```python
from build123d import *

# Parameters (mm, degrees)
F0_W      = 42
F0_H      = 63
F0_R      = 1.75
F0_R_2    = 11.5
F1_DEPTH  = 4
F2_W      = 42
F2_H      = 3
F3_DEPTH  = 30
F4_R      = 2.876713
F4_R_2    = 4.342344
F4_R_3    = 6.646556
F5_DEPTH  = 4
F6_W      = 3
F6_H      = 10
F7_DEPTH  = 10
F8_R      = 2
F9_DEPTH  = 25
F10_W     = 3
F10_H     = 34
F11_DEPTH = 10
F12_R     = 2
F13_DEPTH = 25


with BuildPart() as f1:
    # F0 (on Top) → F1 (new body)
    with BuildSketch(Plane.XY):
        Rectangle(F0_W, F0_H)
        with Locations((-15.5, -5)):
            Circle(F0_R, mode=Mode.SUBTRACT)
        with Locations((15.5, -5)):
            Circle(F0_R, mode=Mode.SUBTRACT)
        with Locations((-15.5, 26)):
            Circle(F0_R, mode=Mode.SUBTRACT)
        with Locations((0, 10.5)):
            Circle(F0_R_2, mode=Mode.SUBTRACT)
        with Locations((15.5, 26)):
            Circle(F0_R, mode=Mode.SUBTRACT)
    extrude(amount=F1_DEPTH)

    # F2 (on face) → F3 (join)
    with BuildSketch(Plane.XY.offset(4)):
        with Locations((0, -30)):
            Rectangle(F2_W, F2_H)
    extrude(amount=F3_DEPTH)

    # F4 (on face) → F5 (join)
    with BuildSketch(Plane(origin=(-21, 0, 0), x_dir=(0, -1, 0), z_dir=(-1, 0, 0))):
        Polygon((28.5, 34), (-31.5, 4), (28.5, 4), align=None)
        with Locations((-5.90477, 9.762893)):
            Circle(F4_R, mode=Mode.SUBTRACT)
        with Locations((4.623126, 12.472619)):
            Circle(F4_R_2, mode=Mode.SUBTRACT)
        with Locations((19.102728, 16.427787)):
            Circle(F4_R_3, mode=Mode.SUBTRACT)
        Polygon((28.5, 4), (-31.5, 4), (-31.5, 0), (31.5, 0), (31.5, 34), (28.5, 34), align=None)
    extrude(amount=F5_DEPTH)

    # F6 (on face) → F7 (join)
    with BuildSketch(Plane.YZ.offset(21)):
        with Locations((-30, 29)):
            Rectangle(F6_W, F6_H)
    extrude(amount=F7_DEPTH)

    # F8 (on face) → F9 (cut)
    with BuildSketch(Plane(origin=(0, -28.5, 0), x_dir=(-1, 0, 0), z_dir=(0, 1, 0))):
        with Locations((-26.502214, 29.595299)):
            Circle(F8_R)
    extrude(amount=-F9_DEPTH, mode=Mode.SUBTRACT)

    # F10 (on face) → F11 (join)
    with BuildSketch(Plane(origin=(-25, 0, 0), x_dir=(0, -1, 0), z_dir=(-1, 0, 0))):
        with Locations((30, 17)):
            Rectangle(F10_W, F10_H)
    extrude(amount=F11_DEPTH)

    # F12 (on face) → F13 (cut)
    with BuildSketch(Plane.XZ.offset(31.5)):
        with Locations((-31, 29)):
            Circle(F12_R)
        with Locations((-31, 5)):
            Circle(F12_R)
    extrude(amount=-F13_DEPTH, mode=Mode.SUBTRACT)


solid = f1.part
```
CAD build for the part. Positions are in the model's coordinates, mm. A direction names the side the tool comes from. Give positions to 0.01 mm unless a question says otherwise; leave off trailing zeros. Write each loop counter-clockwise with the first axis right and the second up, starting at its lowest first coordinate (ties: lowest second). Pieces come first, ordered by that corner, then holes. Notation, with made-up numbers: (-17, 47.25) -> (40, 47.25) arc R22 cw to (40, 64.25) -> close; hole circle Ø4 at (20.25, -17.75). An arc over 180 degrees is marked (long way). Write each question's results on one line, items separated by ' | '.
1. Cut at A-A, the plane y = 10.5. Write the cut outline in (x, z).
Geometry check:
outline: (-25, 0) -> (-11.5, 0) -> (-11.5, 4) -> (-21, 4) -> (-21, 14.5) -> (-25, 14.5) -> close; (11.5, 0) -> (21, 0) -> (21, 4) -> (11.5, 4) -> close
2. Two-plate mould, pull along Y, no slides. Class faces 5 (the flat face through (-30, -28.5, 17)), 6 (the cylindrical face through (-22.972, -1.423, 15.407)), 7 (the cylindrical face through (-22.97, -18.24, 23.02)), 8 (the flat face through (0, -7, 0)): pulls with the +Y half, pulls with the -Y half, needs draft (parallel to the pull), parting line crosses it, or undercut.
Geometry check:
face 5: pulls with the +Y half | face 6: undercut | face 7: undercut | face 8: needs draft
3. Wall check: probe 1 along Y at (x, z) = (-15.5, 2.45); probe 2 along Z at (x, y) = (-31, -30.45); probe 3 along Y at (x, z) = (0, 1.6). Give the ranges that are in metal, low to high. Write a range as [from, to].
Geometry check:
probe 1: [-31.5, -6.75], [-3.25, 24.25], [27.75, 31.5] | probe 2: [0, 3], [7, 27], [31, 34] | probe 3: [-31.5, -1], [22, 31.5]
4. Cut at C-C, the plane x = 0. Write the cut outline in (y, z).
Geometry check:
outline: (-31.5, 0) -> (-1, 0) -> (-1, 4) -> (-28.5, 4) -> (-28.5, 34) -> (-31.5, 34) -> close; (22, 0) -> (31.5, 0) -> (31.5, 4) -> (22, 4) -> close
5. Which spindle directions (+Z, -Z, +X, -X, +Y, -Y) get a long thin tool onto all of the face, cutting with end or side? Do faces 1 (the cylindrical face through (-13.883, -5.67, 1.972)), 2 (the flat face through (21, -5, 3)), 3 (the flat face through (-1, -28.5, 19)), 4 (the flat face through (-25, -5, 6)). Say none if no direction does.
Geometry check:
face 1: +Z, -Z | face 2: -Z, +X, +Y, -Y | face 3: +Z, +X, +Y | face 4: +Z, -Z, -X, +Y
6. Drop flat-ended pins along their axis: P1, Ø12.5, axis at x = 4.5, y = -11, coming from the +Z side; P2, Ø17.5, axis at y = -19.1, z = 16.43, coming from the -X side; P3, Ø10, axis at y = 5.5, z = 8, coming from the +X side. Give the stop position or say it passes through.
Geometry check:
P1: z = 4 | P2: x = -25 | P3: x = 21
7. Cut at B-B, the plane x = -31. Write the cut outline in (y, z), then the cut area to 3 significant figures.
Geometry check:
outline: (-31.5, 0) -> (-28.5, 0) -> (-28.5, 3) -> (-31.5, 3) -> close; (-31.5, 7) -> (-28.5, 7) -> (-28.5, 27) -> (-31.5, 27) -> close; (-31.5, 31) -> (-28.5, 31) -> (-28.5, 34) -> (-31.5, 34) -> close | area: 78.0 mm²
8. Cut at D-D, the plane y = -5. Write the cut outline in (x, z), then the cut area to 3 significant figures.
Geometry check:
outline: (-25, 0) -> (-17.25, 0) -> (-17.25, 4) -> (-21, 4) -> (-21, 8.15) -> (-25, 8.15) -> close; (-25, 16.8) -> (-21, 16.8) -> (-21, 22.25) -> (-25, 22.25) -> close; (-13.75, 0) -> (13.75, 0) -> (13.75, 4) -> (-13.75, 4) -> close; (17.25, 0) -> (21, 0) -> (21, 4) -> (17.25, 4) -> close | area: 194 mm²
